```python
from build123d import *

# Parameters (mm, degrees)
BOSS_EXTRUDE1_DEPTH = 97.5
SHELL2_START        = -95.5
SHELL2_DEPTH        = 191
SHELL2_START_2      = -96
SHELL2_2_DEPTH      = 192


with BuildPart() as part:
    # Sketch2 → Boss-Extrude1 (new, symmetric)
    with BuildSketch(Plane.XY):
        Polygon((0, 100), (245, 45), (280, 0), (0, 0), (-25, 0), (-25, 45), (0, 45), align=None)
    extrude(amount=BOSS_EXTRUDE1_DEPTH, both=True)

    # Shell2: read off the stored shape, not the designer's step
    # Shell2 outline → Shell2 (cut)
    with BuildSketch(Plane.XY.offset(SHELL2_START)):
        Polygon((-25, 45), (-25, 2), (-23.5, 2), (-23.5, 1.5), (276.933040958, 1.5), (276.815971674, 1.650517651), (278, 2.571428571), (245, 45), (2, 99.551020408), (1.671442487, 98.08744603), (1.5, 98.125933119), (1.5, 45), align=None)
    extrude(amount=SHELL2_DEPTH, mode=Mode.SUBTRACT)

    # Shell2 2 outline → Shell2 2 (cut)
    with BuildSketch(Plane.XY.offset(SHELL2_START_2)):
        Polygon((-23.5, 45), (-23.5, 1.5), (276.933040958, 1.5), (244.146362645, 43.654300688), (1.5, 98.125933119), (1.5, 45), align=None)
    extrude(amount=SHELL2_2_DEPTH, mode=Mode.SUBTRACT)


solid = part.part
```
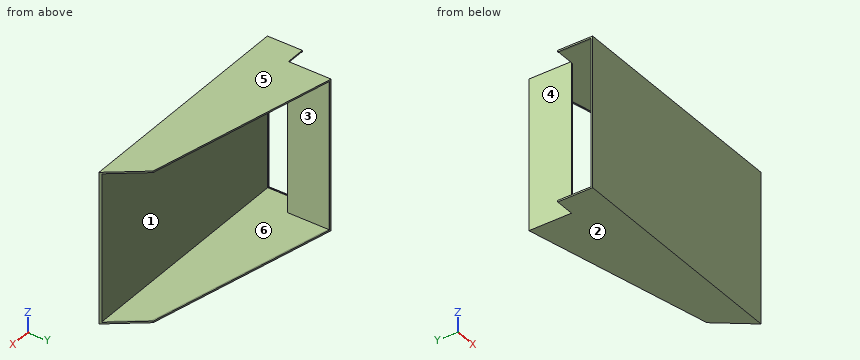
Geometry check sheet. Reference: the model listing, model coordinates, mm. Face numbers are marked on the shaded views. A direction names the side the tool comes from. Round coordinates to 2 decimals unless told otherwise and drop trailing zeros. Write each loop counter-clockwise with the first axis right and the second up, starting at its lowest first coordinate (ties: lowest second). Pieces come first, ordered by that corner, then holes. Notation, with made-up numbers: (23, 7.5) - (41, 7.5) arc R8 cw to (41, 11.5) - close; hole circle Ø9 at (5.5, 17.5). An arc over 180 degrees is marked (long way). Write each question's results on one line, items separated by ' | '.
(1) Sectioned sample at D-D, the plane x = 156. Enter the section's corners in (y, z), plus the area to 3 significant figures.
Computed:
outline: (0, -97.5) - (64.98, -97.5) - (64.98, -95.5) - (63.44, -95.5) - (63.44, -96) - (1.5, -96) - (1.5, 96) - (63.44, 96) - (63.44, 95.5) - (64.98, 95.5) - (64.98, 97.5) - (0, 97.5) - close | area: 484 mm^2
(2) Draft check along Z on the marked faces 1, 2, 3 and 4. Enter one of: pulls with the +Z half, pulls with the -Z half, needs draft (parallel to the pull), parting line crosses it, or undercut.
Computed:
face 1: undercut | face 2: pulls with the -Z half | face 3: undercut | face 4: needs draft
(3) Thickness scan on probe 1 along Z at (x, y) = (59, 13); probe 2 along X at (y, z) = (79.5, 73). Record the ranges inside material, lowest first. Write a range as from..to.
Computed:
probe 1: z = -97.5..-96, 96..97.5 | probe 2: x = 0..1.5
(4) Set-up check for the marked faces 5 and 6: record each of +Z, -Z, +X, -X, +Y, -Y from which the full face is reachable in a straight line by a thin tool's end or side.
Computed:
face 5: +Z, +X, -X, +Y, -Y | face 6: none
(5) Sectioned sample at A-A, the plane z = 46.5. Enter the section's corners in (x, y).
Computed:
outline: (-25, 0) - (280, 0) - (278, 2.57) - (276.82, 1.65) - (276.93, 1.5) - (-23.5, 1.5) - (-23.5, 2) - (-25, 2) - close; (0, 45) - (1.5, 45) - (1.5, 98.13) - (1.67, 98.09) - (2, 99.55) - (0, 100) - close
(6) Depth check by flat-ended pin: pin 1 Ø0.6 at (x, z) = (-10.5, -96.5) entering from +Y; pin 2 Ø5 at (y, z) = (43.5, 73) entering from -X; pin 3 Ø10 at (y, z) = (88.5, -30.5) entering from +X. Enter the tip coordinate at first touch or a pass-through.
Computed:
pin 1: stops at y = 45 | pin 2: stops at x = 0 | pin 3: stops at x = 1.5
(7) Sectioned sample at C-C, the plane y = 59. Enter the section's corners in (x, z).
Computed:
outline: (0, -97.5) - (182.64, -97.5) - (182.64, -95.5) - (175.79, -95.5) - (175.79, -96) - (1.5, -96) - (1.5, 96) - (175.79, 96) - (175.79, 95.5) - (182.64, 95.5) - (182.64, 97.5) - (0, 97.5) - close
(8) Sectioned sample at B-B, the plane y = 31. Enter the section's corners in (x, z).
Computed:
outline: (-25, -97.5) - (255.89, -97.5) - (255.89, -95.5) - (253.99, -95.5) - (253.99, -96) - (-23.5, -96) - (-23.5, -95.5) - (-25, -95.5) - close; (-25, 95.5) - (-23.5, 95.5) - (-23.5, 96) - (253.99, 96) - (253.99, 95.5) - (255.89, 95.5) - (255.89, 97.5) - (-25, 97.5) - close
